The drawing under review shows one solid part. Ordinate dimensions are in mm from its lowest x, y, z. A direction names the side the tool comes from. Round coordinates to 2 decimals unless told otherwise and drop trailing zeros. Order: outer loops, then holes, each group sorted by start corner. A loop starts at its lowest first (then second) coordinate and runs counter-clockwise, first axis right, second up.
1) Consider section D-D (x = 93.5). Give the boundary of the cut face in (y, z), then the cut area to 3 significant figures.
2) To check wall thickness, follow L1, parallel to Z at x = 21.5, y = 3.25; L2, parallel to X at y = 2.5, z = 3 (1 decimal); L3, parallel to X at y = 20.5, z = 12. State the ranges of each line that lie inside material, in increasing order.
3) Mouldability with a two-part tool opening along Z and no side actions: class the marked faces 4, 5 and 6 as pulls with the +Z half, pulls with the -Z half, needs draft (parallel to the pull), parting line crosses it, or undercut.
4) Machinability: for the marked faces 1, 2 and 3, which of the approach directions +Z, -Z, +X, -X, +Y, -Y give a long, thin tool a straight path to every point of the face, cutting with its end or side? Answer none if there is none.
5) Consider section A-A (x = 46). Give the boundary of the cut face in (y, z).
6) Consider section C-C (z = 20.5). Give the boundary of the cut face in (x, y) (1 decimal), then the cut area to 3 significant figures.
7) Clearance check with flat-ended pins moving along their axes: P1, Ø1.9, axis at x = 20.5, y = 1.5, coming from the +Z side; P2, Ø1.5, axis at x = 28.5, z = 49, coming from the +Y side; P3, Ø10.5, axis at y = 19.5, z = 21.5, coming from the +X side. State where each tip first meets the part, or that it passes through.
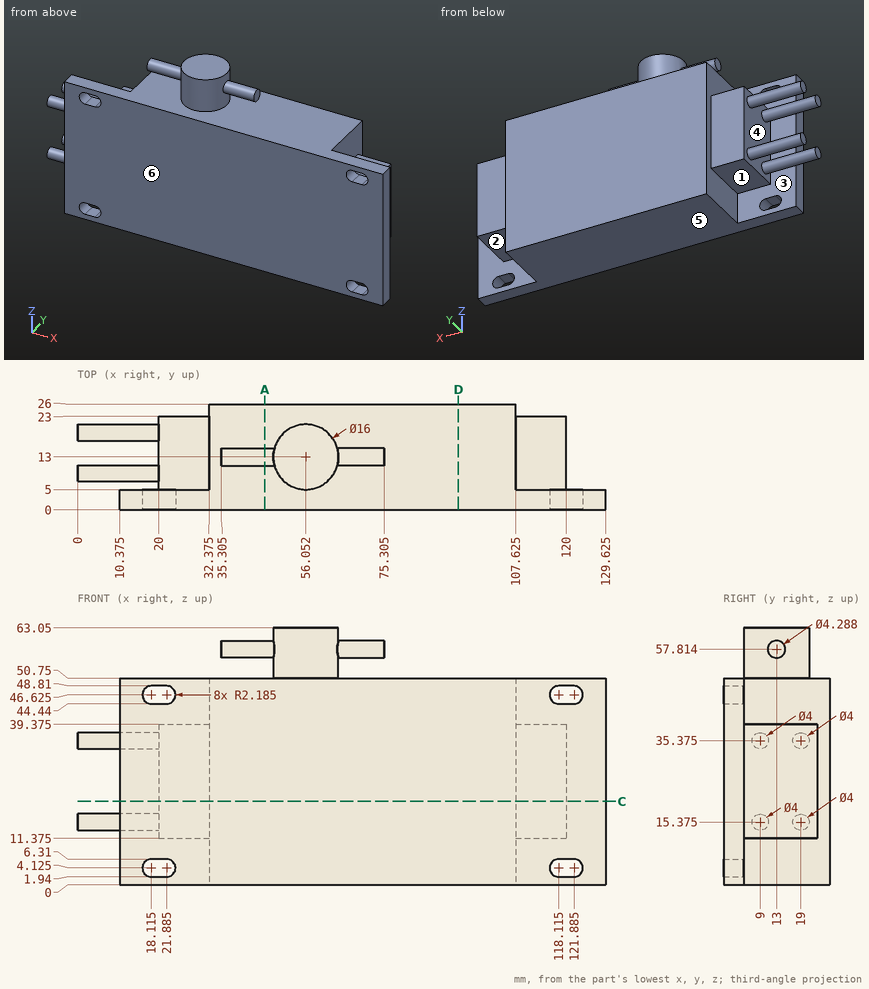
Answer below:
1. outline: (0, 0) - (26, 0) - (26, 50.75) - (0, 50.75) - close
1. area: 1,320 mm2
2. L1: z = 0 to 1.94, 6.31 to 44.44, 48.81 to 50.75
2. L2: x = 10.4 to 16.2, 23.8 to 116.2, 123.8 to 129.6
2. L3: x = 20 to 120
3. face 4: undercut
3. face 5: pulls with the -Z half
3. face 6: needs draft
4. face 1: -Z, -X, +Y
4. face 2: -Z, +X, +Y
4. face 3: -X
5. outline: (0, 0) - (26, 0) - (26, 50.75) - (0, 50.75) - close; circle Ø4.29 at (13, 57.81)
6. outline: (10.4, 0) - (129.6, 0) - (129.6, 5) - (120, 5) - (120, 23) - (107.6, 23) - (107.6, 26) - (32.4, 26) - (32.4, 23) - (20, 23) - (20, 5) - (10.4, 5) - close
6. area: 2,620 mm2
7. P1: stops at z = 50.75
7. P2: stops at y = 5
7. P3: stops at x = 120
